Design review of the part built by this model. Coordinates are the model's own, in mm. A direction names the side the tool comes from. Round coordinates to 2 decimals unless told otherwise and drop trailing zeros. Loops run counter-clockwise (first coordinate to the right, second up) from the corner with the lowest first, then second, coordinate; pieces in that order, holes last. Notation, with made-up numbers: (-9, 41) -> (40, 41) arc R19 ccw to (40, 72) -> close; hole circle Ø9 at (79, 6.25). An arc over 180 degrees is marked (long way). Use a Markdown table: item, result. Add a question column.
from build123d import *

# Parameters (mm, degrees)
SKETCH_3_R          = 2.5
EXTRUDE_1_DEPTH     = 15
SKETCH_4_W          = 25
SKETCH_4_H          = 12
CUT_EXTRUDE_1_DEPTH = 15
SKETCH_1_R          = 35
SKETCH_1_R_2        = 5
SKETCH_1_R_3        = 2.5
EXTRUDE_2_DEPTH     = 3
FILLET_1_R          = 1


with BuildPart() as part:
    # Sketch 3 → Extrude 1 (new, symmetric)
    with BuildSketch(Plane(origin=(0, 0, 0), x_dir=(1, 0, 0), z_dir=(0, 1, 0))):
        with BuildLine():
            Line((-10, 0), (10, 0))
            Line((10, 0), (5.262640911, 15.598314937))
            ThreePointArc((5.262640911, 15.598314937), (0, 19.5), (-5.262640911, 15.598314937))
            Line((-5.262640911, 15.598314937), (-10, 0))
        make_face()
        with Locations(Location((0, 14, 0), (0, 0, 270))):
            Circle(SKETCH_3_R, mode=Mode.SUBTRACT)
    extrude(amount=EXTRUDE_1_DEPTH, both=True)

    # Sketch 4 → Cut-Extrude 1 (cut, symmetric)
    with BuildSketch(Plane(origin=(0, 0, 0), x_dir=(0, 0, -1), z_dir=(1, 0, 0))):
        with Locations((12.5, 0)):
            Rectangle(SKETCH_4_W, SKETCH_4_H)
    extrude(amount=CUT_EXTRUDE_1_DEPTH, both=True, mode=Mode.SUBTRACT)


with BuildPart() as cut_extrude_1_piece_1:
    # of the separate pieces the step leaves, piece 1, a body of its own (cut_extrude_1_pieces)
    add(part.part.solids().sort_by_distance((-10, -6, 0))[0])



with BuildPart() as cut_extrude_1_piece_2:
    # of the separate pieces the step leaves, piece 2, a body of its own (cut_extrude_1_pieces)
    add(part.part.solids().sort_by_distance((-10, 15, 0))[0])


with BuildPart() as cut_extrude_1_piece_1_1:
    add(cut_extrude_1_piece_1.part)

    add(cut_extrude_1_piece_2.part)  # Extrude 2 merges Cut-Extrude 1 piece 2
    # Sketch 1 → Extrude 2 (add)
    with BuildSketch(Plane.XY):
        Circle(SKETCH_1_R)
        Circle(SKETCH_1_R_2, mode=Mode.SUBTRACT)
        with Locations((0, 30)):
            Circle(SKETCH_1_R_3, mode=Mode.SUBTRACT)
        with Locations((15, 25.980762114)):
            Circle(SKETCH_1_R_3, mode=Mode.SUBTRACT)
        with Locations((25.980762114, 15)):
            Circle(SKETCH_1_R_3, mode=Mode.SUBTRACT)
        with Locations((30, 0)):
            Circle(SKETCH_1_R_3, mode=Mode.SUBTRACT)
        with Locations((25.980762114, -15)):
            Circle(SKETCH_1_R_3, mode=Mode.SUBTRACT)
        with Locations((15, -25.980762114)):
            Circle(SKETCH_1_R_3, mode=Mode.SUBTRACT)
        with Locations((0, -30)):
            Circle(SKETCH_1_R_3, mode=Mode.SUBTRACT)
        with Locations((-15, -25.980762114)):
            Circle(SKETCH_1_R_3, mode=Mode.SUBTRACT)
        with Locations((-25.980762114, -15)):
            Circle(SKETCH_1_R_3, mode=Mode.SUBTRACT)
        with Locations((-30, 0)):
            Circle(SKETCH_1_R_3, mode=Mode.SUBTRACT)
        with Locations((-25.980762114, 15)):
            Circle(SKETCH_1_R_3, mode=Mode.SUBTRACT)
        with Locations((-15, 25.980762114)):
            Circle(SKETCH_1_R_3, mode=Mode.SUBTRACT)
    extrude(amount=EXTRUDE_2_DEPTH)

    # Fillet 1
    fillet_1_edges = [cut_extrude_1_piece_1_1.edges().sort_by_distance(p)[0] for p in [
        (-5, 0, 3),
    ]]
    fillet(fillet_1_edges, radius=FILLET_1_R)


solid = cut_extrude_1_piece_1_1.part
1. Consider section A-A on x = 0. Give the number of separate pieces and of enclosed holes in the cut face, plus the area to 3 significant figures.
2. For faces 1 (the face through (0, -6, -7)), 2 (the face through (0, 15, -8)), 3 (the face through (-26.52, 12.56, 1.48)), list the 3-axis set-ups (+Z, -Z, +X, -X, +Y, -Y) from which the entire face can be reached by the end or side of a thin tool; tool diameter is ignored.
3. Consider section B-B on y = 0. State the section outline as (x, z) points, plus the area to 3 significant figures.
4. Consider section C-C on z = -3.75. State the section outline as (x, y) points.
5. Mouldability with a two-part tool opening along Z and no side actions: class faces 4 (the face through (0, -7, 3)), 5 (the face through (0.1, 10.4, -16.5)), 6 (the face through (7.664, -10.437, -7.69)), 7 (the face through (-0.33, -27.52, 1.48)) as +Z half, -Z half, draft (parallel to the pull), parting line (faces both ways), or undercut.
6. To check wall thickness, follow probe 1 along Y at (x, z) = (-4, -14.5); probe 2 along Z at (x, y) = (11, -11); probe 3 along Y at (x, z) = (15, 2.15). State the ranges of each line that lie inside material, in increasing order. Write a range as from..to.
7. Consider section D-D on x = 14.5. State the section outline as (y, z) points, plus the area to 3 significant figures.
8. Insertion check: P1, Ø6, axis at x = -25.98, y = 15, coming from the -Z side; P2, Ø2, axis at x = 2, z = -9, coming from the +Y side; P3, Ø10, axis at x = 4.5, z = -9, coming from the -Y side. Each pin has a flat end and moves straight along its axis. Give the tip position at first contact, or say it passes through.
Verdict:
| question | item | result |
|---|---|---|
| 1 | separate pieces | 6 |
| 1 | enclosed holes | 0 |
| 1 | area | 411 mm² |
| 2 | face 1 | -Z, +X, -X |
| 2 | face 2 | -Z, +X, -X, +Y |
| 2 | face 3 | +Z, -Z |
| 3 | outline | (-35, 0) -> (-32.5, 0) -> (-32.5, 3) -> (-35, 3) -> close; (-27.5, 0) -> (-5, 0) -> (-5, 2) arc R1 ccw to (-6, 3) -> (-27.5, 3) -> close; (5, 0) -> (27.5, 0) -> (27.5, 3) -> (6, 3) arc R1 ccw to (5, 2) -> close; (32.5, 0) -> (35, 0) -> (35, 3) -> (32.5, 3) -> close |
| 3 | area | 150 mm² |
| 4 | outline | (-8.86, -15) -> (8.86, -15) -> (8.86, -6) -> (-8.86, -6) -> close; (-8.86, 6) -> (8.86, 6) -> (8.86, 15) -> (-8.86, 15) -> close |
| 5 | face 4 | +Z half |
| 5 | face 5 | undercut |
| 5 | face 6 | -Z half |
| 5 | face 7 | draft |
| 6 | probe 1 | y = -15..-6, 6..15 |
| 6 | probe 2 | z = 0..3 |
| 6 | probe 3 | y = -31.62..-28.48, -23.48..23.48, 28.48..31.62 |
| 7 | outline | (-31.86, 0) -> (-28.43, 0) -> (-28.43, 3) -> (-31.86, 3) -> close; (-23.53, 0) -> (23.53, 0) -> (23.53, 3) -> (-23.53, 3) -> close; (28.43, 0) -> (31.86, 0) -> (31.86, 3) -> (28.43, 3) -> close |
| 7 | area | 162 mm² |
| 8 | P1 | stops at z = 0 |
| 8 | P2 | stops at y = 15 |
| 8 | P3 | stops at y = -15 |
